```python
from build123d import *

# Parameters (mm, degrees)
SKETCH1_W           = 60
SKETCH1_H           = 30
SKETCH1_R           = 1.6
BOSS_EXTRUDE1_DEPTH = 2
SKETCH2_W           = 2
SKETCH2_H           = 19
BOSS_EXTRUDE2_DEPTH = 4
SKETCH3_W           = 2
SKETCH3_H           = 13
BOSS_EXTRUDE3_DEPTH = 10
SKETCH4_W           = 5.906565556
SKETCH4_H           = 2.906405273
SKETCH4_W_2         = 2.156365203
SKETCH4_H_2         = 1.218815115
BOSS_EXTRUDE4_DEPTH = 1
BOSS_EXTRUDE5_DEPTH = 8
SKETCH7_W           = 3
SKETCH7_H           = 3
CUT_EXTRUDE1_DEPTH  = 9
SKETCH9_W           = 1
SKETCH9_H           = 1
CUT_EXTRUDE2_DEPTH  = 9


with BuildPart() as part:
    # Sketch1 → Boss-Extrude1 (new body)
    with BuildSketch(Plane(origin=(0, 0, 0), x_dir=(1, 0, 0), z_dir=(0, 1, 0))):
        with Locations((30, 15)):
            Rectangle(SKETCH1_W, SKETCH1_H)
        with Locations(Location((4, 4, 0), (0, 0, 270))):
            Circle(SKETCH1_R, mode=Mode.SUBTRACT)
        with Locations(Location((4, 26, 0), (0, 0, 90))):
            Circle(SKETCH1_R, mode=Mode.SUBTRACT)
        with Locations(Location((56, 26, 0), (0, 0, 270))):
            Circle(SKETCH1_R, mode=Mode.SUBTRACT)
        with Locations(Location((56, 4, 0), (0, 0, 90))):
            Circle(SKETCH1_R, mode=Mode.SUBTRACT)
    extrude(amount=BOSS_EXTRUDE1_DEPTH)

    # Sketch2 → Boss-Extrude2 (add)
    with BuildSketch(Plane(origin=(0, 2, 0), x_dir=(1, 0, 0), z_dir=(0, 1, 0))):
        with Locations((25.5, 16.5)):
            Rectangle(SKETCH2_W, SKETCH2_H)
        with Locations((47.5, 16.5)):
            Rectangle(SKETCH2_W, SKETCH2_H)
    extrude(amount=BOSS_EXTRUDE2_DEPTH)

    # Sketch3 → Boss-Extrude3 (add)
    with BuildSketch(Plane(origin=(0, 2, 0), x_dir=(1, 0, 0), z_dir=(0, 1, 0))):
        with Locations((53.405190381, 12.053258952)):
            Rectangle(SKETCH3_W, SKETCH3_H)
    extrude(amount=BOSS_EXTRUDE3_DEPTH)

    # Sketch4 → Boss-Extrude4 (add)
    with BuildSketch(Plane(origin=(0, 2, 0), x_dir=(1, 0, 0), z_dir=(0, 1, 0))):
        with Locations((18.796276446, 24.187990865)):
            Rectangle(SKETCH4_W, SKETCH4_H)
        with Locations((15.514851138, 8.530904392)):
            Rectangle(SKETCH4_W_2, SKETCH4_H_2)
    extrude(amount=BOSS_EXTRUDE4_DEPTH)

    # Sketch6 → Boss-Extrude5 (add)
    with BuildSketch(Plane(origin=(0, 2, 0), x_dir=(1, 0, 0), z_dir=(0, 1, 0))):
        Polygon((9, 23), (9, 15), (0, 15), (-1, 16), (-1, 22), (0, 23), align=None)
    extrude(amount=BOSS_EXTRUDE5_DEPTH)

    # Sketch7 → Cut-Extrude1 (cut)
    with BuildSketch(Plane.ZY.offset(1)):
        with Locations((-19, 7.75)):
            Rectangle(SKETCH7_W, SKETCH7_H)
        with Locations((-19, 4.25)):
            Rectangle(SKETCH7_W, SKETCH7_H)
    extrude(amount=-CUT_EXTRUDE1_DEPTH, mode=Mode.SUBTRACT)

    # Sketch9 → Cut-Extrude2 (cut)
    with BuildSketch(Plane(origin=(0, 12, 0), x_dir=(1, 0, 0), z_dir=(0, 1, 0))):
        with Locations((53.405190381, 13.053258952)):
            Rectangle(SKETCH9_W, SKETCH9_H)
        with Locations((53.405190381, 17.053258952)):
            Rectangle(SKETCH9_W, SKETCH9_H)
        with Locations((53.405190381, 15.053258952)):
            Rectangle(SKETCH9_W, SKETCH9_H)
        with Locations((53.405190381, 11.053258952)):
            Rectangle(SKETCH9_W, SKETCH9_H)
        with Locations((53.405190381, 9.053258952)):
            Rectangle(SKETCH9_W, SKETCH9_H)
        with Locations((53.405190381, 7.053258952)):
            Rectangle(SKETCH9_W, SKETCH9_H)
    extrude(amount=-CUT_EXTRUDE2_DEPTH, mode=Mode.SUBTRACT)


solid = part.part
```
Geometry check sheet. Reference: the model listing, model coordinates, mm. A direction names the side the tool comes from. Coordinates: 2 decimals unless noted, no trailing zeros. Order: outer loops, then holes, each group sorted by start corner. A loop starts at its lowest first (then second) coordinate and runs counter-clockwise, first axis right, second up. Notation, with made-up numbers: M -38.75,54.25 L 1.25,54.25 A4 ccw 1.25,59.25 Z; hole C 4.25,33 d9. An arc over 180 degrees is marked long. One line per question, with ' | ' between items. Start each with the question number.
Item 1: Cross-section at B-B on x = 4. Enter the section's corners in (y, z), then the cut area to 3 significant figures.
Item 2: Set-up check for faces 4 (the flat face through (4, 10, -19)), 5 (the flat face through (0, 1, -15)), 6 (the flat face through (26.5, 4, -16)), 7 (the flat face through (3, 2.75, -19)): record each of +Z, -Z, +X, -X, +Y, -Y from which the full face is reachable in a straight line by a thin tool's end or side.
Item 3: Material ranges on L1, parallel to X at y = 4.25, z = -13; L2, parallel to X at y = 1.1, z = -26; L3, parallel to X at y = 6.25, z = -9, recorded low to high. Write a range as [from, to].
Item 4: Cross-section at C-C on x = 56. Enter the section's corners in (y, z).
Item 5: Cross-section at A-A on z = -4. Enter the section's corners in (x, y).
Item 6: Gauge pin test, flat ends, axial feed: pin 1 (0.6 mm diameter, centred on x = 53, y = 5.5, fed in from -Z); pin 2 (1 mm diameter, centred on x = 48, y = 5, fed in from -Z); pin 3 (2 mm diameter, centred on y = 1.5, z = -26.5, fed in from -X). Record the tip position at first contact, or that the pin passes through.
Item 7: Cross-section at D-D on y = 8.25. State how many separate pieces and enclosed holes the cut face has, then the cut area to 3 significant figures.
Item 8: Draft check along Z on faces 1 (the flat face through (60, 1, -15)), 2 (the flat face through (3, 4, -20.5)), 3 (the flat face through (53, 7, -18.553)). Enter one of: pulls with the +Z half, pulls with the -Z half, needs draft (parallel to the pull), parting line crosses it, or undercut.
Findings:
1) outline: M 0,-30 L 2,-30 L 2,-27.6 L 0,-27.6 Z; M 0,-24.4 L 2,-24.4 L 2,-23 L 10,-23 L 10,-15 L 2,-15 L 2,-5.6 L 0,-5.6 Z; M 0,-2.4 L 2,-2.4 L 2,0 L 0,0 Z; hole M 2.75,-20.5 L 5.75,-20.5 L 5.75,-17.5 L 2.75,-17.5 Z; hole M 6.25,-20.5 L 9.25,-20.5 L 9.25,-17.5 L 6.25,-17.5 Z | area: 93.2 mm²
2) face 4: +Z, -Z, -X, +Y | face 5: +Z, -Z, -X, -Y | face 6: +Z, -Z, +Y | face 7: -X
3) L1: x = [24.5, 26.5], [46.5, 48.5], [52.41, 52.91], [53.91, 54.41] | L2: x = [0, 2.4], [5.6, 54.4], [57.6, 60] | L3: x = [52.41, 52.91], [53.91, 54.41]
4) outline: M 0,-30 L 2,-30 L 2,-27.6 L 0,-27.6 Z; M 0,-24.4 L 2,-24.4 L 2,-5.6 L 0,-5.6 Z; M 0,-2.4 L 2,-2.4 L 2,0 L 0,0 Z
5) outline: M 0,0 L 2.4,0 L 2.4,2 L 0,2 Z; M 5.6,0 L 54.4,0 L 54.4,2 L 5.6,2 Z; M 57.6,0 L 60,0 L 60,2 L 57.6,2 Z
6) pin 1: stops at z = -18.55 | pin 2: stops at z = -26 | pin 3: stops at x = 0
7) separate pieces: 2 | enclosed holes: 6 | area: 72.0 mm²
8) face 1: needs draft | face 2: undercut | face 3: pulls with the -Z half
